Verification items for the finished model (mm, model axes). Face numbers are marked on the shaded views. A direction names the side the tool comes from. Give positions to 0.01 mm unless a question says otherwise; leave off trailing zeros. Loops run counter-clockwise (first coordinate to the right, second up) from the corner with the lowest first, then second, coordinate; pieces in that order, holes last. Notation, with made-up numbers: M 22.25,5.5 L 58.25,5.5 A17 cw 58.25,38.5 Z; hole C 34,47.25 d10. An arc over 180 degrees is marked long. Answer in a Markdown table with one row per item.
```python
from build123d import *

# Parameters (mm, degrees)
CROQUIS1_W              = 30
CROQUIS1_H              = 33
SALIENTE_EXTRUIR1_DEPTH = 22
CROQUIS2_R              = 2
SALIENTE_EXTRUIR2_DEPTH = 8
CHAFL_N1_SIZE           = 5
CHAFL_N2_SIZE           = 5
CROQUIS3_R              = 2
CORTAR_EXTRUIR1_DEPTH   = 35


with BuildPart() as part:
    # Croquis1 → Saliente-Extruir1 (new body)
    with BuildSketch(Plane.XY):
        with Locations((-0.166051661, -4.433579336)):
            Rectangle(CROQUIS1_W, CROQUIS1_H)
    extrude(amount=SALIENTE_EXTRUIR1_DEPTH)

    # Croquis2 → Saliente-Extruir2 (add)
    with BuildSketch(Plane.XY.offset(22)):
        with Locations((-6.416051661, -10.933579336)):
            Circle(CROQUIS2_R)
        with Locations((6.083948339, -10.933579336)):
            Circle(CROQUIS2_R)
    extrude(amount=SALIENTE_EXTRUIR2_DEPTH)

    # Chaflán1
    chafl_n1_edges = [part.edges().sort_by_distance(p)[0] for p in [
        (-0.166051661, 12.066420664, 0),
    ]]
    chamfer(chafl_n1_edges, length=CHAFL_N1_SIZE)

    # Chaflán2
    chafl_n2_edges = [part.edges().sort_by_distance(p)[0] for p in [
        (-0.166051661, -20.933579336, 0),
    ]]
    chamfer(chafl_n2_edges, length=CHAFL_N2_SIZE)

    # Croquis3 → Cortar-Extruir1 (cut)
    with BuildSketch(Plane(origin=(14.833948339, 0, 0), x_dir=(0, 0, -1), z_dir=(1, 0, 0))):
        with Locations(Location((-12, 2.066420664, 0), (0, 0, 90))):
            Circle(CROQUIS3_R)
    extrude(amount=-CORTAR_EXTRUIR1_DEPTH, mode=Mode.SUBTRACT)


solid = part.part
```
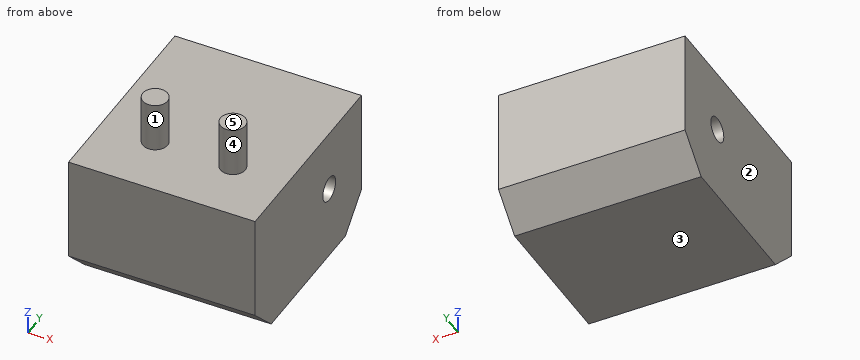
Item 1: Go/stop test with flat-tipped pins: pin 1 (10 mm diameter, centred on x = -5.5, y = -17.5, fed in from +Z); pin 2 (4 mm diameter, centred on x = 7, y = 6.5, fed in from +Z). Record where each tip stops, or that it passes through.
Reported:
| item | result |
|---|---|
| pin 1 | stops at z = 30 |
| pin 2 | stops at z = 22 |
Item 2: Tool access check on the marked faces 4 and 5. Record the directions out of +Z, -Z, +X, -X, +Y, -Y that give a thin tool (end or side, any length) a straight path to the whole face; none if there is none.
Reported:
| item | result |
|---|---|
| face 4 | +Z |
| face 5 | +Z, +X, -X, +Y, -Y |
Item 3: Sectioned sample at B-B (x = -10.5). Record the cut outline in (y, z), and give its area (3 significant figures).
Reported:
| item | result |
|---|---|
| outline | M -20.93,5 L -15.93,0 L 7.07,0 L 12.07,5 L 12.07,22 L -20.93,22 Z; hole C 2.07,12 d4 |
| area | 688 mm^2 |
Item 4: Sectioned sample at C-C (y = 3). Record the cut outline in (x, z).
Reported:
| item | result |
|---|---|
| outline | M -15.17,0 L 14.83,0 L 14.83,10.23 L -15.17,10.23 Z; M -15.17,13.77 L 14.83,13.77 L 14.83,22 L -15.17,22 Z |
Item 5: Scan lines: L1, parallel to Z at x = -0.25, y = 5; L2, parallel to Y at x = 11.75, z = 13.5; L3, parallel to Z at x = 12.25, y = 2.5. Record each from-to range of solid material in increasing order. Write a range as [from, to].
Reported:
| item | result |
|---|---|
| L1 | z = [0, 22] |
| L2 | y = [-20.93, 0.74], [3.39, 12.07] |
| L3 | z = [0, 10.05], [13.95, 22] |
Item 6: Sectioned sample at D-D (y = -12). Record the cut outline in (x, z), and give its area (3 significant figures).
Reported:
| item | result |
|---|---|
| outline | M -15.17,0 L 14.83,0 L 14.83,22 L 7.78,22 L 7.78,30 L 4.39,30 L 4.39,22 L -4.72,22 L -4.72,30 L -8.11,30 L -8.11,22 L -15.17,22 Z |
| area | 714 mm^2 |
Item 7: Release check for a two-part mould opening along X. For the marked faces 1, 2 and 3 record: released by +X, released by -X, zero draft, split by the parting line, or undercut.
Reported:
| item | result |
|---|---|
| face 1 | undercut |
| face 2 | released by -X |
| face 3 | zero draft |
Item 8: Sectioned sample at A-A (z = 12). Record the cut outline in (x, y).
Reported:
| item | result |
|---|---|
| outline | M -15.17,-20.93 L 14.83,-20.93 L 14.83,0.07 L -15.17,0.07 Z; M -15.17,4.07 L 14.83,4.07 L 14.83,12.07 L -15.17,12.07 Z |
